Could you check a few things on this drawing? It's one solid part, dimensions in mm from its lowest x, y, z. A direction names the side the tool comes from. Coordinates: 2 decimals unless noted, no trailing zeros. Order: outer loops, then holes, each group sorted by start corner. A loop starts at its lowest first (then second) coordinate and runs counter-clockwise, first axis right, second up.
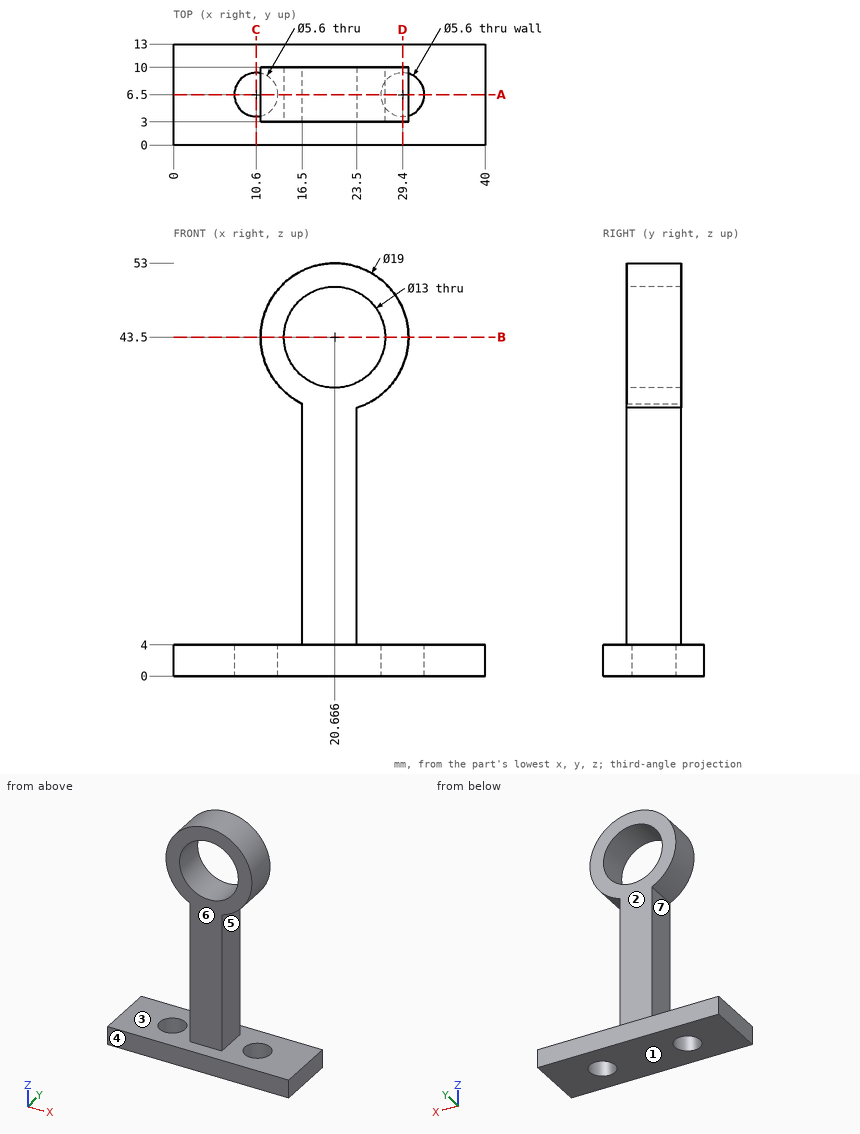
1. Imagine slicing it at B-B on z = 43.5. Please give me the cut outline in (x, y), then the cut area to 3 significant figures.
Completed:
outline: (11.17, 3) - (14.17, 3) - (14.17, 10) - (11.17, 10) - close; (27.17, 3) - (30.17, 3) - (30.17, 10) - (27.17, 10) - close
area: 42.0 mm2
2. On a 3-axis mill with a long thin cutter (end or side, diameter ignored), from which of +Z, -Z, +X, -X, +Y, -Y can I reach the whole of each face in a straight line? I mean the marked faces 4, 5, 6 and 7. Say none if no direction works.
Completed:
face 4: +Z, -Z, +X, -X, -Y
face 5: +X, +Y, -Y
face 6: +Z, +X, -X, -Y
face 7: -X, +Y, -Y
3. Imagine slicing it at D-D on x = 29.4. Please give me the cut outline in (y, z).
Completed:
outline: (0, 0) - (3.7, 0) - (3.7, 4) - (0, 4) - close; (3, 39.76) - (10, 39.76) - (10, 47.24) - (3, 47.24) - close; (9.3, 0) - (13, 0) - (13, 4) - (9.3, 4) - close
4. Imagine slicing it at C-C on x = 10.6. Please give me the cut outline in (y, z), then the cut area to 3 significant figures.
Completed:
outline: (0, 0) - (3.7, 0) - (3.7, 4) - (0, 4) - close; (9.3, 0) - (13, 0) - (13, 4) - (9.3, 4) - close
area: 29.6 mm2
5. Thinking about a two-plate mould opening in Z: for the marked faces 1, 2 and 3, which applies, pulls with the +Z half, pulls with the -Z half, needs draft (parallel to the pull), parting line crosses it, or undercut?
Completed:
face 1: pulls with the -Z half
face 2: needs draft
face 3: undercut
6. Imagine slicing it at A-A on y = 6.5. Please give me the cut outline in (x, z).
Completed:
outline: (0, 0) - (7.8, 0) - (7.8, 4) - (0, 4) - close; (13.4, 0) - (26.6, 0) - (26.6, 4) - (23.5, 4) - (23.5, 34.43) arc R9.5 ccw (long way) to (16.5, 34.96) - (16.5, 4) - (13.4, 4) - close; (32.2, 0) - (40, 0) - (40, 4) - (32.2, 4) - close; hole circle Ø13 at (20.67, 43.5)
7. I'm going to push flat-ended pins straight in: pin 1 (5 mm diameter, centred on x = 28, y = 6, fed in from -Z); pin 2 (4.5 mm diameter, centred on x = 29.4, y = 6.5, fed in from +Z); pin 3 (5 mm diameter, centred on x = 6, y = 10, fed in from +Z); pin 4 (5.5 mm diameter, centred on x = 16.5, z = 22.5, fed in from -Y). Where does each tip first touch, or does it pass through?
Completed:
pin 1: stops at z = 0
pin 2: stops at z = 50.44
pin 3: stops at z = 4
pin 4: stops at y = 3
8. Please list where these lines run through material, in increasing order: probe 1 along X at (y, z) = (7.5, 43.5); probe 2 along Z at (x, y) = (26, 4.75) (1 decimal); probe 3 along Y at (x, z) = (10.6, 1.7).
Completed:
probe 1: x = 11.17 to 14.17, 27.17 to 30.17
probe 2: z = 0 to 4, 35.6 to 39.8, 47.2 to 51.4
probe 3: y = 0 to 3.7, 9.3 to 13
